Verification items for the finished model (mm, model axes). Face numbers are marked on the shaded views. A direction names the side the tool comes from. Round coordinates to 2 decimals unless told otherwise and drop trailing zeros. Write each loop counter-clockwise with the first axis right and the second up, starting at its lowest first coordinate (ties: lowest second). Pieces come first, ordered by that corner, then holes. Notation, with made-up numbers: (8.25, 19) - (41.25, 19) arc R19 cw to (41.25, 42) - close; hole circle Ø11 at (70.25, 27.5). An arc over 180 degrees is marked (long way). Answer as a JSON object with one key per item and string values.
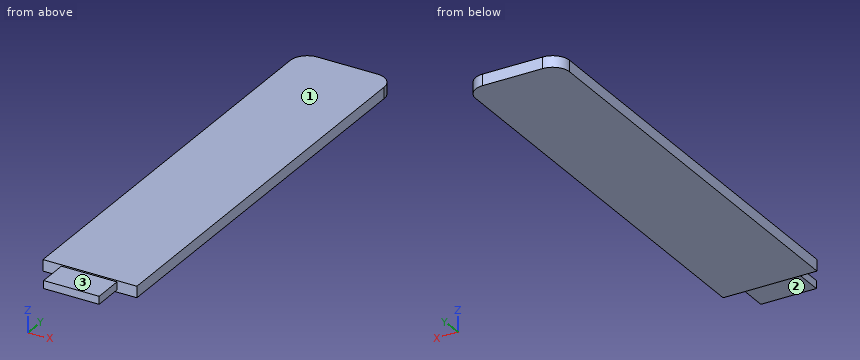
```python
from build123d import *

# Parameters (mm, degrees)
F1_DEPTH = 1.524
F2_R     = 2.286
F3_W     = 7.501836
F3_H     = 1.057486
F4_DEPTH = 4.064


with BuildPart() as f1:
    # F0 (on Top) → F1 (new body)
    with BuildSketch(Plane.XY):
        Polygon((-6.250669, 49.563318), (-6.250669, -8.998585), (-4.305575, -8.998585), (4.510465, -8.998585), (6.438088, -8.998585), (6.438088, 49.563318), align=None)
    extrude(amount=F1_DEPTH)

    # F2
    f2_edges = [f1.edges().sort_by_distance(p)[0] for p in [
        (-6.250669, 49.563318, 0.762),
        (6.438088, 49.563318, 0.762),
    ]]
    fillet(f2_edges, radius=F2_R)

    # F3 (on face) → F4 (join)
    with BuildSketch(Plane.XZ.offset(8.998585)):
        with Locations((0, 0.820748)):
            Rectangle(F3_W, F3_H)
    extrude(amount=F4_DEPTH)


solid = f1.part
```
1. Cross-section at A-A (x = -1.25). Record the boundary of the cut face in (y, z), plus the area to 3 significant figures.
Completed:
{"outline": "(-13.06, 0.29) - (-9, 0.29) - (-9, 0) - (49.56, 0) - (49.56, 1.52) - (-9, 1.52) - (-9, 1.35) - (-13.06, 1.35) - close", "area": "93.5 mm^2"}
2. Cross-section at C-C (x = -4.5). Record the boundary of the cut face in (y, z), plus the area to 3 significant figures.
Completed:
{"outline": "(-9, 0) - (49.5, 0) - (49.5, 1.52) - (-9, 1.52) - close", "area": "89.2 mm^2"}
3. Material ranges on probe 1 along Y at (x, z) = (3, 1.45); probe 2 along Y at (x, z) = (-5.5, 0.2), recorded low to high. Write a range as from..to.
Completed:
{"probe 1": "y = -9..49.56", "probe 2": "y = -9..48.97"}
4. Go/stop test with a flat-tipped pin: pin 1 (4.5 mm diameter, centred on x = 0, y = -11.5, fed in from +Z). Record where the tip stops, or that it passes through.
Completed:
{"pin 1": "stops at z = 1.35"}
5. Cross-section at B-B (z = 0.7). Record the boundary of the cut face in (x, y).
Completed:
{"outline": "(-6.25, -9) - (-3.75, -9) - (-3.75, -13.06) - (3.75, -13.06) - (3.75, -9) - (6.44, -9) - (6.44, 47.28) arc R2.29 ccw to (4.15, 49.56) - (-3.96, 49.56) arc R2.29 ccw to (-6.25, 47.28) - close"}
6. Access from +Z, -Z, +X, -X, +Y, -Y to the whole of each face (thin tool, end or side, straight path). Record for the marked faces 1, 2 and 3.
Completed:
{"face 1": "+Z, +X, -X, +Y, -Y", "face 2": "-Z, +X, -X, -Y", "face 3": "+Z, +X, -X, -Y"}
